Design review of the part built by this model. Coordinates are the model's own, in mm. Round coordinates to 2 decimals unless told otherwise and drop trailing zeros. Write each loop counter-clockwise with the first axis right and the second up, starting at its lowest first coordinate (ties: lowest second). Pieces come first, ordered by that corner, then holes. Notation, with made-up numbers: M -20,-31.75 L 11,-31.75 A17 cw 11,-2.75 Z; hole C 44,66 d9. An arc over 180 degrees is marked long. One line per question, with ' | ' between items. Start each with the question number.
Item 1: Draft analysis for pull direction Z (two halves, no side actions). For faces 1 (the face through (-37, 0, -33)), 2 (the face through (0.355, 0.74, -56.088)), state which applies: released by +Z, released by -Z, zero draft, split by the parting line, or undercut.
Item 2: Add section A-A, the plane z = -58. State the section outline as (x, y) points.
Item 3: For L1, parallel to X at y = 0.85, z = -47.5; L2, parallel to X at y = 0.7, z = -10; L3, parallel to Z at x = 0.5, y = 0.6, list the stretches that pass through material, from the lowest coordinate up.
Autodesk Inventor part; units mm, degrees
ref_plane "YZ Plane" through (0, 0, 0) normal (1, 0, 0) x (0, 1, 0)
ref_plane "XZ Plane" through (0, 0, 0) normal (0, 1, 0) x (-1, 0, 0)
ref_plane "XY Plane" through (0, 0, 0) normal (0, 0, 1) x (1, 0, 0)
sketch "スケッチ1" plane through (0, 0, 0) normal (0, 1, 0) x (-1, 0, 0)
  line L0 (-20.4773, 9.5578) -> (96.5227, 9.5578)
  line L1 (96.5227, 9.5578) -> (96.5227, -77.4422)
  line L2 (96.5227, -77.4422) -> (-20.4773, -77.4422)
  line L3 (-20.4773, -77.4422) -> (-20.4773, 9.5578)
  point P0 (0, 0)
  dimension "d0" = 117
  dimension "d1" = 87
extrude "押し出し1" add sketch "スケッチ1" along normal blind 1.5
sketch "スケッチ2" plane through (0, 1.5, 0) normal (0, 1, 0) x (1, 0, 0)
  line L0 (-96.5227, -9.5578) -> (20.4773, -9.5578)
  line L1 (20.4773, -9.5578) -> (20.4773, 77.4422)
  line L2 (20.4773, 77.4422) -> (-96.5227, 77.4422)
  line L3 (-96.5227, 77.4422) -> (-96.5227, -9.5578)
  point P0 (0, 0)
  point P1 (-76.5227, 72.4422)
  point P2 (0.4773, 72.4422)
  point P3 (-76.5227, -4.5578)
  point P4 (0.4773, -4.5578)
  dimension "d4" = 5
  dimension "d5" = 5
  dimension "d6" = 5
  dimension "d7" = 5
  dimension "d8" = 20
  dimension "d9" = 20
  dimension "d10" = 20
  dimension "d11" = 20
hole "穴1" at (-76.5227, 1.5, -72.4422) at (0.4773, 1.5, -72.4422) at (-76.5227, 1.5, 4.5578) at (0.4773, 1.5, 4.5578) direction (0, -1, 0) diameter 3 end through all
sketch "スケッチ3" plane through (0, 1.5, 0) normal (0, 1, 0) x (1, 0, 0)
  line L0 (-96.5227, -9.5578) -> (20.4773, -9.5578)
  line L1 (20.4773, -9.5578) -> (20.4773, 77.4422)
  line L2 (20.4773, 77.4422) -> (-96.5227, 77.4422)
  line L3 (-96.5227, 77.4422) -> (-96.5227, -9.5578)
  point P0 (0, 0)
  point P1 (-91.5227, 47.4422)
  point P2 (-91.5227, 47.4422)
  point P3 (-91.5227, 62.4422)
  point P4 (-91.5227, 20.4422)
  point P5 (-91.5227, 5.4422)
  point P6 (15.4773, 62.4422)
  point P7 (15.4773, 47.4422)
  point P8 (15.4773, 20.4422)
  point P9 (15.4773, 5.4422)
  dimension "d19" = 5
  dimension "d20" = 5
  dimension "d21" = 5
  dimension "d22" = 5
  dimension "d23" = 30
  dimension "d24" = 15
  dimension "d25" = 15
  dimension "d26" = 30
  dimension "d27" = 15
  dimension "d28" = 30
  dimension "d29" = 15
  dimension "d30" = 30
  dimension "d31" = 5
  dimension "d32" = 5
  dimension "d33" = 5
  dimension "d34" = 5
hole "穴2" at (-91.5227, 1.5, -47.4422) at (-91.5227, 1.5, -62.4422) at (-91.5227, 1.5, -20.4422) at (-91.5227, 1.5, -5.4422) at (15.4773, 1.5, -62.4422) at (15.4773, 1.5, -47.4422) at (15.4773, 1.5, -20.4422) at (15.4773, 1.5, -5.4422) direction (0, -1, 0) diameter 3 end through all
sketch "スケッチ4" plane through (0, 1.5, 0) normal (0, 1, 0) x (1, 0, 0)
  line L0 (20.4773, -9.5578) -> (20.4773, 77.4422)
  line L1 (20.4773, 77.4422) -> (-96.5227, 77.4422)
  line L2 (5.1573, 61.2472) -> (-81.2027, 61.2472)
  line L3 (-81.2027, 61.2472) -> (-81.2027, 6.6372)
  line L4 (-81.2027, 61.2472) -> (5.1573, 61.2472)
  line L5 (5.1573, 6.6372) -> (-81.2027, 6.6372)
  line L6 (-81.2027, 6.6372) -> (-81.2027, 61.2472)
  line L7 (-81.2027, 6.6372) -> (5.1573, 6.6372)
  line L8 (5.1573, 6.6372) -> (5.1573, 61.2472)
  point P0 (-96.5227, -9.5578)
  point P1 (0, 0)
  point P2 (0, 0)
  point P3 (0, 0)
  point P4 (-0.5577, 54.8972)
  point P5 (-0.5577, 12.9872)
  point P6 (-66.5977, 9.8122)
  point P7 (-66.5977, 58.0722)
  dimension "d42" = 86.36
  dimension "d43" = 54.61
  dimension "d44" = 14.605
  dimension "d45" = 3.175
  dimension "d46" = 3.175
  dimension "d47" = 14.605
  dimension "d48" = 6.35
  dimension "d50" = 6.35
  dimension "d52" = 0
  dimension "d53" = 0
  dimension "d54" = 87
  dimension "d55" = 16.195
  dimension "d56" = 117
  dimension "d58" = 15.32
  dimension "d59" = 5.715
  dimension "d60" = 5.715
  dimension "d61" = 66.04
  dimension "d62" = 66.04
hole "穴3" at (-66.5977, 1.5, -58.0722) at (-66.5977, 1.5, -9.8122) at (-0.5577, 1.5, -12.9872) at (-0.5577, 1.5, -54.8972) direction (0, -1, 0) diameter 3 end through all
equation "\"d55\" = 0.5 * d54 - 0.5 * d43"
equation "\"d58\" = 0.5 * d56 - 0.5 * d42"
properties part number "バッテリー固定"
Computed values:
1) face 1: zero draft | face 2: undercut
2) outline: M -96.52,0 L -68.1,0 L -68.1,1.5 L -96.52,1.5 Z; M -65.1,0 L 20.48,0 L 20.48,1.5 L -65.1,1.5 Z
3) L1: x = -96.52 to -93.02, -90.02 to 13.98, 16.98 to 20.48 | L2: x = -96.52 to -68.09, -65.11 to 20.48 | L3: z = -77.44 to -73.94, -70.94 to -55.96, -53.83 to -14.05, -11.92 to 3.06, 6.06 to 9.56
